Answer from the drawing. Dimensions are ordinates in mm from the lowest x, y and z of the part. A direction names the side the tool comes from. Coordinates: 2 decimals unless noted, no trailing zeros. Order: outer loops, then holes, each group sorted by start corner. A loop starts at its lowest first (then second) coordinate and runs counter-clockwise, first axis right, second up. Notation, with made-up numbers: (-7, 10) - (20, 10) arc R17 cw to (20, 38) - close; hole circle Ø5 at (-8, 15.25). An arc over 180 degrees is marked (long way). One line per item, written item: value. Start each with the question number.
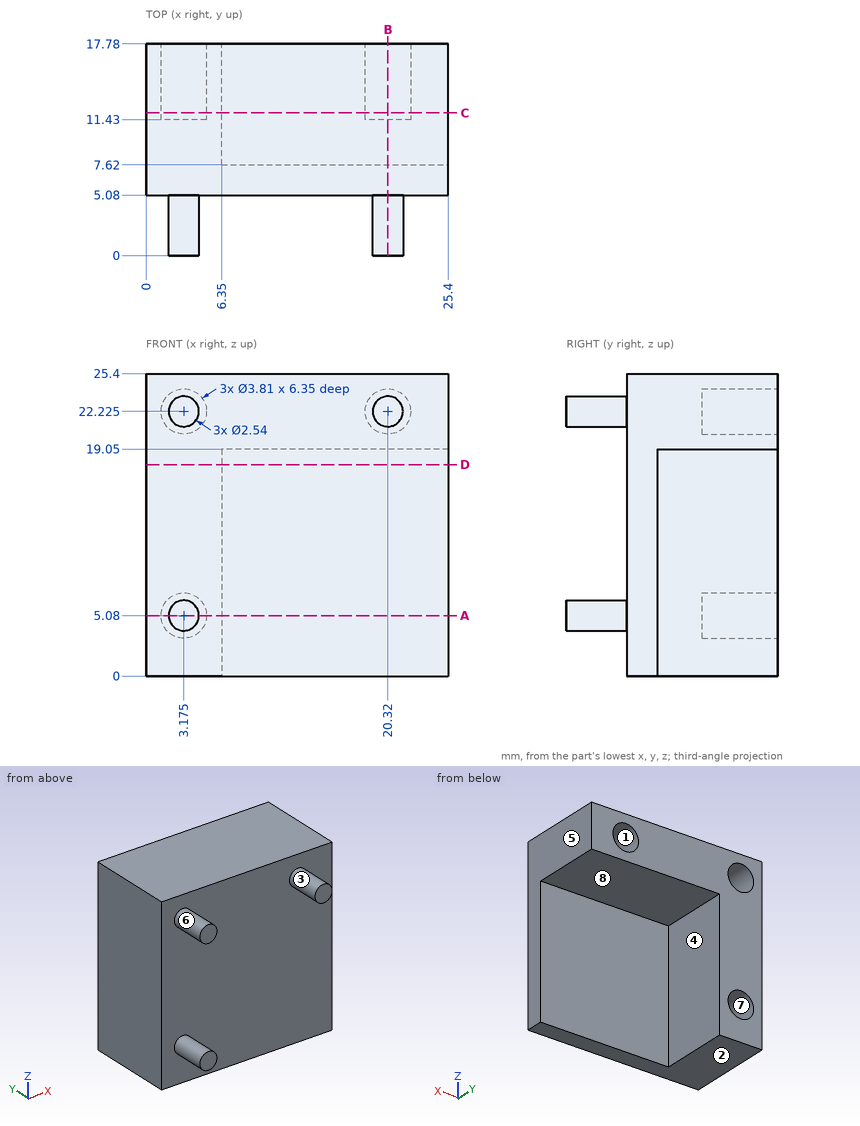
(1) For the marked faces 1, 2, 3 and 4, determine the directions among +Z, -Z, +X, -X, +Y, -Y from which every point of the face is accessible in a straight line to the end or side of a thin tool.
(2) The part is cut by section A-A on z = 5.08. Determine the outline of the cut face in (x, y) (3 decimals), plus the area to 3 significant figures.
(3) For a pull along Z with two mould halves and no side action, classify the marked faces 5, 6, 7 and 8 as pulls with the +Z half, pulls with the -Z half, needs draft (parallel to the pull), parting line crosses it, or undercut.
(4) Consider probe 1 along Z at (x, y) = (20.32, 16.5); probe 2 along X at (y, z) = (13, 20.5); probe 3 along X at (y, z) = (8, 12.25). Determine where each line is inside the solid, lowest interval first.
(5) Flat-ended cylindrical pins translate along their axes: pin 1 Ø4 at (x, y) = (17, 5) entering from -Z; pin 2 Ø1.1 at (x, z) = (2.5, 5) entering from +Y; pin 3 Ø10 at (x, z) = (14, 21) entering from -Y; pin 4 Ø8 at (y, z) = (13.5, 8) entering from +X. Find the tip coordinate at first contact, or state that the pin passes through.
(6) The part is cut by section D-D on z = 17.75. Determine the outline of the cut face in (x, y), plus the area to 3 significant figures.
(7) The part is cut by section B-B on x = 20.32. Determine the outline of the cut face in (y, z) (3 decimals), plus the area to 3 significant figures.
(8) The part is cut by section C-C on y = 12. Determine the outline of the cut face in (x, z) (3 decimals).
Completed:
1. face 1: +Y
1. face 2: -Z, +X, -X, +Y, -Y
1. face 3: -Y
1. face 4: -Z, +X, +Y
2. outline: (0, 5.08) - (1.905, 5.08) - (1.905, 0) - (4.445, 0) - (4.445, 5.08) - (25.4, 5.08) - (25.4, 7.62) - (6.35, 7.62) - (6.35, 17.78) - (5.08, 17.78) - (5.08, 11.43) - (1.27, 11.43) - (1.27, 17.78) - (0, 17.78) - close
2. area: 118 mm2
3. face 5: needs draft
3. face 6: undercut
3. face 7: undercut
3. face 8: pulls with the -Z half
4. probe 1: z = 19.05 to 20.32, 24.13 to 25.4
4. probe 2: x = 0 to 2.37, 3.98 to 19.51, 21.13 to 25.4
4. probe 3: x = 0 to 6.35
5. pin 1: stops at z = 0
5. pin 2: stops at y = 11.43
5. pin 3: stops at y = 5.08
5. pin 4: stops at x = 6.35
6. outline: (0, 5.08) - (25.4, 5.08) - (25.4, 7.62) - (6.35, 7.62) - (6.35, 17.78) - (0, 17.78) - close
6. area: 129 mm2
7. outline: (0, 20.955) - (5.08, 20.955) - (5.08, 0) - (7.62, 0) - (7.62, 19.05) - (17.78, 19.05) - (17.78, 20.32) - (11.43, 20.32) - (11.43, 24.13) - (17.78, 24.13) - (17.78, 25.4) - (5.08, 25.4) - (5.08, 23.495) - (0, 23.495) - close
7. area: 118 mm2
8. outline: (0, 0) - (6.35, 0) - (6.35, 19.05) - (25.4, 19.05) - (25.4, 25.4) - (0, 25.4) - close; hole circle Ø3.81 at (3.175, 5.08); hole circle Ø3.81 at (3.175, 22.225); hole circle Ø3.81 at (20.32, 22.225)
